```python
from build123d import *

# Parameters (mm, degrees)
SKETCH1_W           = 37
SKETCH1_H           = 7.63
SKETCH1_R           = 1.2
BOSS_EXTRUDE1_DEPTH = 0.44


with BuildPart() as part:
    # Sketch1 → Boss-Extrude1 (new body)
    with BuildSketch(Plane.XY):
        Rectangle(SKETCH1_W, SKETCH1_H)
        with Locations((-14.59410802, 0)):
            Circle(SKETCH1_R, mode=Mode.SUBTRACT)
        with Locations((15.15, 0)):
            Circle(SKETCH1_R, mode=Mode.SUBTRACT)
    extrude(amount=BOSS_EXTRUDE1_DEPTH)

    # Sketch2 → Revolve2 (revolve)
    with BuildSketch(Plane(origin=(0, 0, 0), x_dir=(1, 0, 0), z_dir=(0, 1, 0))):
        with BuildLine():
            Line((0, 0), (0, 4.42))
            ThreePointArc((0, 4.42), (-1.543186446, 3.522040816), (-1.525, 1.736704894))
            Line((-1.525, 1.736704894), (-1.525, 0))
            Line((-1.525, 0), (0, 0))
        make_face()
    revolve(axis=Axis((0, 0, 0), (0, 0, -1)))


solid = part.part
```
Verification items for the finished model (mm, model axes). Round coordinates to 2 decimals unless told otherwise and drop trailing zeros. Order: outer loops, then holes, each group sorted by start corner. A loop starts at its lowest first (then second) coordinate and runs counter-clockwise, first axis right, second up. Notation, with made-up numbers: (-34.75, 79) -> (-12.75, 79) arc R21 ccw to (-12.75, 95) -> close; hole circle Ø3 at (47.5, 78). An arc over 180 degrees is marked (long way). Put each result on its own line as item: value. Start each with the question number.
(1) Section check C-C (x = 0). Enter the section's corners in (y, z) (3 decimals), then the cut area to 3 significant figures.
(2) Draft check along X on faces 1 (the face through (1.524, 0.067, -0.856)), 2 (the face through (16.26, -0.46, 0.22)), 3 (the face through (0, -2, 0)). Enter one of: +X half, -X half, draft (parallel to the pull), parting line (faces both ways), or undercut.
(3) Material ranges on line 1 along Y through (x, z) = (15.15, 0.1) (3 decimals); line 2 along Z through (x, y) = (-12.5, 1.5); line 3 along X through (y, z) = (-1, 0.15), recorded low to high.
(4) Section check B-B (y = 0). Enter the section's corners in (x, z) (3 decimals).
(5) Section check A-A (x = 15.15). Enter the section's corners in (y, z) (3 decimals).
(6) Depth check by flat-ended pin: pin 1 Ø1.9 at (x, y) = (-14.59, 0) entering from +Z; pin 2 Ø2 at (y, z) = (0, -3) entering from -X (3 decimals); pin 3 Ø3 at (x, y) = (3.5, -1) entering from -Z; pin 4 Ø1.5 at (x, z) = (0, -0.5) entering from -Y (3 decimals). Enter the tip coordinate at first touch or a pass-through.
(7) Section check D-D (z = -0.65). Enter the section's corners in (x, y) (3 decimals).
Completed:
1. outline: (-3.815, 0) -> (-1.525, 0) -> (-1.525, -1.737) arc R1.775 ccw (long way) to (1.525, -1.737) -> (1.525, 0) -> (3.815, 0) -> (3.815, 0.44) -> (-3.815, 0.44) -> close
1. area: 16.7 mm2
2. face 1: parting line
2. face 2: undercut
2. face 3: draft
3. line 1: y = -3.815 to -1.2, 1.2 to 3.815
3. line 2: z = 0 to 0.44
3. line 3: x = -18.5 to -15.26, -13.93 to 14.49, 15.81 to 18.5
4. outline: (-18.5, 0) -> (-15.794, 0) -> (-15.794, 0.44) -> (-18.5, 0.44) -> close; (-13.394, 0) -> (-1.525, 0) -> (-1.525, -1.737) arc R1.775 ccw (long way) to (1.525, -1.737) -> (1.525, 0) -> (13.95, 0) -> (13.95, 0.44) -> (-13.394, 0.44) -> close; (16.35, 0) -> (18.5, 0) -> (18.5, 0.44) -> (16.35, 0.44) -> close
5. outline: (-3.815, 0) -> (-1.2, 0) -> (-1.2, 0.44) -> (-3.815, 0.44) -> close; (1.2, 0) -> (3.815, 0) -> (3.815, 0.44) -> (1.2, 0.44) -> close
6. pin 1: passes through
6. pin 2: stops at x = -1.775
6. pin 3: stops at z = 0
6. pin 4: stops at y = -3.815
7. outline: circle Ø3.05 at (0, 0)
